Part model, mm, in its own coordinate system. Round coordinates to 2 decimals unless told otherwise and drop trailing zeros. Loops run counter-clockwise (first coordinate to the right, second up) from the corner with the lowest first, then second, coordinate; pieces in that order, holes last. Notation, with made-up numbers: M -2.5,-12 L 25.5,-12 A27 cw 25.5,23 Z; hole C 28.5,44 d6. An arc over 180 degrees is marked long. Put each result on its own line as item: value. Start each with the question number.
1) Slice it at B-B on z = 22. Give the cut face in (x, y).
2) Pull direction X, two halves, no side cores. Call faces 1 (the flat face through (48.13, 54.09, 8.74)), 2 (the flat face through (38, 43, 2)), 3 (the cylindrical face through (4.79, 3.84, 34.62)): +X half, -X half, draft (parallel to the pull), parting line (faces both ways), or undercut.
3) Slice it at C-C on y = 48. Give the cut face in (x, z), then the cut area to 3 significant figures.
4) Probe line 1 along Z through (x, y) = (45, 51.5); line 2 along X through (y, z) = (29, 13); line 3 along Y through (x, z) = (67, -28). List the from-to ranges inside material, lowest first.
5) Slice it at A-A on x = 43. Give the cut face in (y, z), then the cut area to 3 significant figures.
6) Slice it at D-D on x = 23.5. Give the cut face in (y, z).
7) Drop flat-ended pins along their axis: pin 1 Ø6 at (x, z) = (64, 22) entering from +Y; pin 2 Ø6 at (x, z) = (77.5, 15) entering from +Y; pin 3 Ø1 at (y, z) = (48, 7.5) entering from -X. Give the stop position or say it passes through.
```python
from build123d import *

# Parameters (mm, degrees)
ESTRUSIONE_SOTTILE1_DEPTH      = 37
ESTRUSIONE_SOTTILE1_DEPTH_BACK = 37
SCHIZZO2_R                     = 1.7
TAGLIO_ESTRUSIONE2_DEPTH       = 23
SCHIZZO4_W                     = 19
SCHIZZO4_H                     = 35
TAGLIO_ESTRUSIONE4_DEPTH       = 9
SCHIZZO5_R                     = 1.7
TAGLIO_ESTRUSIONE5_DEPTH       = 9
TAGLIO_ESTRUSIONE6_DEPTH       = 38
TAGLIO_ESTRUSIONE6_DEPTH_BACK  = 38


with BuildPart() as part:
    # Schizzo1 → Estrusione-Sottile1 (new body, two sides)
    with BuildSketch(Plane.XY) as estrusione_sottile1_sk:
        with BuildLine():
            Line((1.3418419, 31.371953403), (-14.62198067, 12.132505153))
            Line((-14.62198067, 12.132505153), (0, 0))
            Line((0, 0), (92.590170907, 111.588799848))
            ThreePointArc((92.590170907, 111.588799848), (116.785428363, 124.808829232), (140.980685819, 111.588799848))
            Line((140.980685819, 111.588799848), (138.876827802, 110.238325322))
            ThreePointArc((138.876827802, 110.238325322), (116.710841454, 122.30872327), (94.613803758, 110.112560659))
            Line((94.613803758, 110.112560659), (0.327562568, -3.520327082))
            Line((0.327562568, -3.520327082), (-18.142307752, 11.804942585))
            Line((-18.142307752, 11.804942585), (-0.582102925, 32.96833566))
            Line((-0.582102925, 32.96833566), (1.3418419, 31.371953403))
        make_face()
    extrude(amount=ESTRUSIONE_SOTTILE1_DEPTH)
    extrude(estrusione_sottile1_sk.sketch, amount=-ESTRUSIONE_SOTTILE1_DEPTH_BACK)

    # Schizzo2 → Taglio-Estrusione2 (cut)
    with BuildSketch(Plane(origin=(1.923944825, -1.596382257, 0), x_dir=(0, 0, -1), z_dir=(0.76957793, -0.638552903, 0))):
        with Locations((-6.552412565, 139.86942204)):
            Circle(SCHIZZO2_R)
        with Locations((-6.552412565, 129.05255699)):
            Circle(SCHIZZO2_R)
        with Locations((1.452296176, 134.71047302)):
            Circle(SCHIZZO2_R)
        with Locations((9.457004918, 129.55152401)):
            Circle(SCHIZZO2_R)
        with Locations((1.553386665, 123.82845624)):
            Circle(SCHIZZO2_R)
        with Locations((9.659185895, 118.60435549)):
            Circle(SCHIZZO2_R)
    extrude(amount=-TAGLIO_ESTRUSIONE2_DEPTH, mode=Mode.SUBTRACT)

    # Schizzo4 → Taglio-Estrusione4 (cut)
    with BuildSketch(Plane(origin=(0, 0, 0), x_dir=(0, 0, 1), z_dir=(-0.76957793, 0.638552903, 0))):
        with Locations((-7.5, 57.5)):
            Rectangle(SCHIZZO4_W, SCHIZZO4_H)
    extrude(amount=-TAGLIO_ESTRUSIONE4_DEPTH, mode=Mode.SUBTRACT)

    # Schizzo5 → Taglio-Estrusione5 (cut)
    with BuildSketch(Plane(origin=(0, 0, 0), x_dir=(0, 0, 1), z_dir=(-0.76957793, 0.638552903, 0))):
        with Locations((33, 5.5)):
            Circle(SCHIZZO5_R)
        with Locations((-33, 5.5)):
            Circle(SCHIZZO5_R)
        with Locations((-2, 5.5)):
            Circle(SCHIZZO5_R)
    extrude(amount=-TAGLIO_ESTRUSIONE5_DEPTH, mode=Mode.SUBTRACT)

    # Schizzo6 → Taglio-Estrusione6 (cut, two sides)
    with BuildSketch(Plane.XY) as taglio_estrusione6_sk:
        Polygon((0, 0), (-2.515119204, -3.03119792), (-24.654006172, 16.441396342), (100.036117815, 158.204765097), (192.825186497, 76.590730526), (160.291370892, 39.602209292), (94.613803758, 110.112560659), (92.590170907, 111.588799848), (78.649981188, 114.87986373), align=None)
    extrude(amount=TAGLIO_ESTRUSIONE6_DEPTH, mode=Mode.SUBTRACT)
    extrude(taglio_estrusione6_sk.sketch, amount=-TAGLIO_ESTRUSIONE6_DEPTH_BACK, mode=Mode.SUBTRACT)


solid = part.part
```
Recorded:
1. outline: M -1.6,-1.92 L 0.33,-3.52 L 94.61,110.11 L 92.59,111.59 Z
2. face 1: +X half
2. face 2: draft
2. face 3: undercut
3. outline: M 39.83,-37 L 43.08,-37 L 43.08,-17 L 39.83,-17 Z; M 39.83,2 L 43.08,2 L 43.08,37 L 39.83,37 Z
3. area: 179 mm2
4. line 1: z = -37 to -17, 2 to 37
4. line 2: x = 24.06 to 27.31
4. line 3: y = 76.83 to 80.75
5. outline: M 47.91,-37 L 51.82,-37 L 51.82,-17 L 47.91,-17 Z; M 47.91,2 L 51.82,2 L 51.82,37 L 47.91,37 Z
5. area: 215 mm2
6. outline: M 24.41,-37 L 28.32,-37 L 28.32,37 L 24.41,37 Z
7. pin 1: stops at y = 80.75
7. pin 2: stops at y = 97.02
7. pin 3: stops at x = 39.41
